Read the model definition and answer for the solid it produces. Units are mm, in the model's axes. Coordinates: 2 decimals unless noted, no trailing zeros. Loops run counter-clockwise (first coordinate to the right, second up) from the corner with the lowest first, then second, coordinate; pieces in that order, holes last. Notation, with made-up numbers: (5.25, 76) - (63.25, 76) arc R15 ccw to (63.25, 102) - close; hole circle Ø3 at (-33.5, 0). An arc over 180 degrees is marked (long way). Use one line per item in the form item = value.
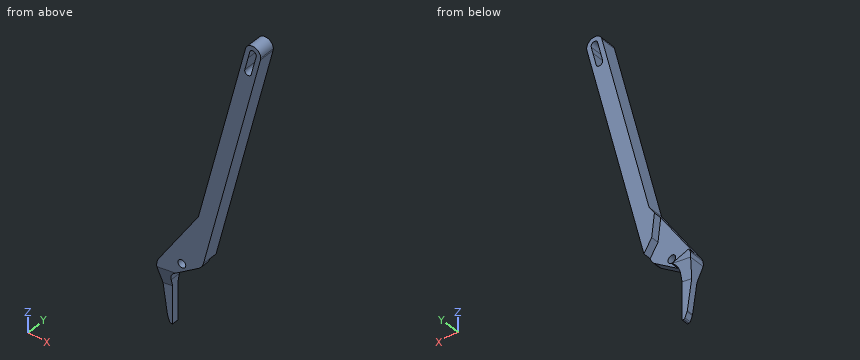
from build123d import *

# Parameters (mm, degrees)
SKETCH1_R           = 3
BOSS_EXTRUDE2_DEPTH = 12
SKETCH3_W           = 12.000133412
SKETCH3_H           = 3.5
CUT_EXTRUDE1_DEPTH  = 214.167200314
CUT_EXTRUDE4_DEPTH  = 6


with BuildPart() as part:
    # Sketch1 → Boss-Extrude2 (new body)
    # profile 1 of 5: a face of its own
    with BuildSketch(Plane(origin=(0, 0, 0), x_dir=(1, 0, 0), z_dir=(0, 1, 0))):
        with BuildLine():
            Line((-19.125338302, 7.287833106), (4.566615153, -9.301451298))
            Line((4.566615153, -9.301451298), (12.801336755, -42.329115693))
            Line((12.801336755, -42.329115693), (49.322165839, -188.806160659))
            ThreePointArc((49.322165839, -188.806160659), (49.451500057, -185.458284048), (51.355769549, -182.701698688))
            Line((51.355769549, -182.701698688), (48.798935765, -172.446798499))
            ThreePointArc((48.798935765, -172.446798499), (50.656289033, -169.355643563), (53.747443969, -171.212996831))
            Line((53.747443969, -171.212996831), (56.304277753, -181.467897021))
            ThreePointArc((56.304277753, -181.467897021), (59.279786353, -183.007817055), (60.965714554, -185.903097912))
            Line((60.965714554, -185.903097912), (16.76676248, -8.630783649))
            ThreePointArc((16.76676248, -8.630783649), (15.305067103, -5.385940236), (12.79956958, -2.858482162))
            Line((12.79956958, -2.858482162), (-5.735764364, 10.120098389))
            ThreePointArc((-5.735764364, 10.120098389), (-8.870108332, 13.694132699), (-10, 18.311618831))
            Line((-10, 18.311618831), (-10, 52.855948326))
            ThreePointArc((-10, 52.855948326), (-10.073223305, 53.032725021), (-10.25, 53.105948326))
            Line((-10.25, 53.105948326), (-11.322967039, 53.105948326))
            ThreePointArc((-11.322967039, 53.105948326), (-11.883595848, 52.934015556), (-12.251443729, 52.477339002))
            Line((-12.251443729, 52.477339002), (-13.870086592, 48.430731845))
            ThreePointArc((-13.870086592, 48.430731845), (-13.980381666, 48.100636263), (-14.05170411, 47.759988049))
            Line((-14.05170411, 47.759988049), (-19.445744306, 11.667622342))
            ThreePointArc((-19.445744306, 11.667622342), (-19.528933908, 9.459922198), (-19.125338302, 7.287833106))
        make_face()
        with Locations(Location((0, 0, 0), (0, 0, 270))):
            Circle(SKETCH1_R, mode=Mode.SUBTRACT)
    # profile 2 of 5: a face of its own
    with BuildSketch(Plane(origin=(0, 0, 0), x_dir=(1, 0, 0), z_dir=(0, 1, 0))):
        with BuildLine():
            ThreePointArc((51.355769549, -182.701698688), (49.451500057, -185.458284048), (49.322165839, -188.806160659))
            Line((49.322165839, -188.806160659), (52.669686095, -187.971530119))
            Line((52.669686095, -187.971530119), (51.355769549, -182.701698688))
        make_face()
    # profile 3 of 5: a face of its own
    with BuildSketch(Plane(origin=(0, 0, 0), x_dir=(1, 0, 0), z_dir=(0, 1, 0))):
        with BuildLine():
            Line((56.304277753, -181.467897021), (57.618194299, -186.737728452))
            Line((57.618194299, -186.737728452), (60.965714554, -185.903097912))
            ThreePointArc((60.965714554, -185.903097912), (59.279786353, -183.007817055), (56.304277753, -181.467897021))
        make_face()
    # profile 4 of 5: a face of its own
    with BuildSketch(Plane(origin=(0, 0, 0), x_dir=(1, 0, 0), z_dir=(0, 1, 0))):
        with BuildLine():
            Line((52.669686095, -187.971530119), (49.322165839, -188.806160659))
            ThreePointArc((49.322165839, -188.806160659), (55.875156257, -193.309906195), (61.143940197, -187.354629285))
            ThreePointArc((61.143940197, -187.354629285), (61.099217106, -186.623413225), (60.965714554, -185.903097912))
            Line((60.965714554, -185.903097912), (57.618194299, -186.737728452))
            ThreePointArc((57.618194299, -186.737728452), (55.76084103, -189.828883387), (52.669686095, -187.971530119))
        make_face()
    # profile 5 of 5: a face of its own
    with BuildSketch(Plane(origin=(0, 0, 0), x_dir=(1, 0, 0), z_dir=(0, 1, 0))):
        with BuildLine():
            Line((12.801336755, -42.329115693), (4.566615153, -9.301451298))
            Line((4.566615153, -9.301451298), (-19.125338302, 7.287833106))
            ThreePointArc((-19.125338302, 7.287833106), (-18.618024546, 5.961975552), (-17.928078586, 4.721314409))
            Line((-17.928078586, 4.721314409), (12.801336755, -42.329115693))
        make_face()
    extrude(amount=BOSS_EXTRUDE2_DEPTH)

    # Sketch3 → Cut-Extrude1 (cut, through all)
    with BuildSketch(Plane(origin=(-20.726542351, 0, -3.097602509), x_dir=(-0.14780941112960405, 0, 0.9890158633619178), z_dir=(-0.9890158633619179, 0, -0.14780941112960405))):
        Polygon((-45.158411705, 0), (-8.665199569, 0), (-22.158545117, 3.5), (-45.158411705, 3.5), align=None)
        Polygon((-22.158545117, 8.5), (-8.665199569, 12), (-45.158411705, 12), (-45.158411705, 8.5), align=None)
        with Locations((-51.158478411, 10.25)):
            Rectangle(SKETCH3_W, SKETCH3_H)
        with Locations((-51.158478411, 1.75)):
            Rectangle(SKETCH3_W, SKETCH3_H)
    extrude(amount=-CUT_EXTRUDE1_DEPTH, mode=Mode.SUBTRACT)

    # Sketch4 → Cut-Extrude4 (cut)
    with BuildSketch(Plane(origin=(0, 12, 0), x_dir=(1, 0, 0), z_dir=(0, 1, 0))):
        Polygon((-4.825296228, 9.482581737), (-17.928078586, 4.721314409), (8.620757021, -35.928145405), (10.712004266, -18.156650248), (16.76676248, -8.630783649), (17.432158169, -2.976226879), align=None)
    extrude(amount=-CUT_EXTRUDE4_DEPTH, mode=Mode.SUBTRACT)


solid = part.part
Item 1: The part is cut by section D-D on x = 32.5. Give the vertices of the cut face in (y, z).
Results below:
outline = (0, 71.73) - (12, 71.73) - (12, 121.34) - (0, 121.34) - close
Item 2: Each of these flat-tipped pins is pushed along its axis until it touches: P1, Ø1.5, axis at x = -2.5, y = 3, coming from the +Z side; P2, Ø1.5, axis at y = 3.5, z = 75, coming from the +X side; P3, Ø10.5, axis at x = 0.5, z = 11.5, coming from the +Y side. Where does it stop, or does it pass through?
Results below:
P1 = 20.05
P2 = 33.5
P3 = 6
Item 3: The part is cut by section A-A on x = 0. Give the vertices of the cut face in (y, z).
Results below:
outline = (0, -6.1) - (6, -6.1) - (6, -3) - (0, -3) - close; (0, 3) - (6, 3) - (6, 22.73) - (0, 22.73) - close
Item 4: The part is cut by section B-B on z = 0. Give the vertices of the cut face in (x, y), plus the area to 3 significant figures.
Results below:
outline = (-14.84, 0) - (-3, 0) - (-3, 6) - (-14.84, 6) - close; (3, 0) - (8.72, 0) - (8.72, 6) - (3, 6) - close
area = 105 mm²
Item 5: Find the intervals of material crossed by L1, parallel to X at y = 1.3, z = 0; L2, parallel to Z at x = 0, y = 2.4; L3, parallel to Z at x = -0.5, y = 3, in increasing order.
Results below:
L1 = -14.84 to -3, 3 to 8.72
L2 = -6.1 to -3, 3 to 22.73
L3 = -6.45 to -2.96, 2.96 to 21.96
Item 6: The part is cut by section C-C on z = 82. Give the vertices of the cut face in (x, y).
Results below:
outline = (22.69, 0) - (35.06, 0) - (35.06, 12) - (22.69, 12) - close
